```python
from build123d import *

# Parameters (mm, degrees)
SKETCH2_W                  = 20.32
SKETCH2_H                  = 2.41
BOSS_EXTRUDE1_DEPTH        = 8.51
SKETCH5_W                  = 1
SKETCH5_H                  = 1
CUT_EXTRUDE1_DEPTH         = 5
CHAMFER1_SIZE              = 0.5
LPATTERN3_COUNT            = 8
LPATTERN3_PITCH            = 2.54
CHAMFER1_OF_LPATTERN3_SIZE = 0.5
SKETCH11_W                 = 0.64
SKETCH11_H                 = 0.64
BOSS_EXTRUDE2_DEPTH        = 9.92
LPATTERN4_COUNT            = 8
LPATTERN4_PITCH            = 2.54


with BuildPart() as part:
    # Sketch2 → Boss-Extrude1 (new body)
    with BuildSketch(Plane(origin=(0, 0, 0), x_dir=(1, 0, 0), z_dir=(0, 1, 0))):
        with Locations((8.89, 0)):
            Rectangle(SKETCH2_W, SKETCH2_H)
    extrude(amount=BOSS_EXTRUDE1_DEPTH)

    # Sketch5 → Cut-Extrude1 (cut)
    with BuildSketch(Plane(origin=(0, 8.51, 0), x_dir=(1, 0, 0), z_dir=(0, 1, 0))):
        Rectangle(SKETCH5_W, SKETCH5_H)
    cut_extrude1 = extrude(amount=-CUT_EXTRUDE1_DEPTH, mode=Mode.SUBTRACT)

    # Chamfer1
    chamfer1_edges = [part.edges().sort_by_distance(p)[0] for p in [
        (0.5, 8.51, 0),
        (0, 8.51, -0.5),
        (-0.5, 8.51, 0),
        (0, 8.51, 0.5),
    ]]
    chamfer(chamfer1_edges, length=CHAMFER1_SIZE)

    # LPattern3: Cut-Extrude1 ×8
    with Locations(*[(i * LPATTERN3_PITCH, 0, 0) for i in range(1, LPATTERN3_COUNT)]):
        add(cut_extrude1, mode=Mode.SUBTRACT)

    # Chamfer1 of LPattern3
    chamfer1_of_lpattern3_edges = [part.edges().sort_by_distance(p)[0] for p in [
        (3.04, 8.51, 0),
        (2.54, 8.51, -0.5),
        (2.04, 8.51, 0),
        (2.54, 8.51, 0.5),
        (5.58, 8.51, 0),
        (5.08, 8.51, -0.5),
        (4.58, 8.51, 0),
        (5.08, 8.51, 0.5),
        (8.12, 8.51, 0),
        (7.62, 8.51, -0.5),
        (7.12, 8.51, 0),
        (7.62, 8.51, 0.5),
        (10.66, 8.51, 0),
        (10.16, 8.51, -0.5),
        (9.66, 8.51, 0),
        (10.16, 8.51, 0.5),
        (13.2, 8.51, 0),
        (12.7, 8.51, -0.5),
        (12.2, 8.51, 0),
        (12.7, 8.51, 0.5),
        (15.74, 8.51, 0),
        (15.24, 8.51, -0.5),
        (14.74, 8.51, 0),
        (15.24, 8.51, 0.5),
        (18.28, 8.51, 0),
        (17.78, 8.51, -0.5),
        (17.28, 8.51, 0),
        (17.78, 8.51, 0.5),
    ]]
    chamfer(chamfer1_of_lpattern3_edges, length=CHAMFER1_OF_LPATTERN3_SIZE)

    # Sketch11 → Boss-Extrude2 (add)
    with BuildSketch(Plane.XZ):
        Rectangle(SKETCH11_W, SKETCH11_H)
    boss_extrude2 = extrude(amount=BOSS_EXTRUDE2_DEPTH)

    # Sketch13 → Loft1 section 0
    with BuildSketch(Plane.XZ.offset(9.92)):
        with BuildLine():
            Line((0.32, -0.32), (0.32, 0.32))
            Line((0.32, 0.32), (-0.32, 0.32))
            Line((-0.32, 0.32), (-0.32, -0.32))
            Line((-0.32, -0.32), (0.32, -0.32))
        make_face()
    # Sketch14 → Loft1 section 1
    with BuildSketch(Plane(origin=(0, -10.49, 0), x_dir=(-1, 0, 0), z_dir=(0, -1, 0))):
        with BuildLine():
            Line((-0.22, 0.22), (0.22, 0.22))
            Line((0.22, 0.22), (0.22, -0.22))
            Line((0.22, -0.22), (-0.22, -0.22))
            Line((-0.22, -0.22), (-0.22, 0.22))
        make_face()
    loft1 = loft()

    # LPattern4: Boss-Extrude2, Loft1 ×8
    with Locations(*[(i * LPATTERN4_PITCH, 0, 0) for i in range(1, LPATTERN4_COUNT)]):
        add(boss_extrude2)
        add(loft1)


solid = part.part
```
Source: CAD feature listing. Evaluate the final solid. Frame: model axes, mm. A direction names the side the tool comes from. Coordinates: 2 decimals unless noted, no trailing zeros. Loops run counter-clockwise (first coordinate to the right, second up) from the corner with the lowest first, then second, coordinate; pieces in that order, holes last. Notation, with made-up numbers: M 65.5,15 L 100.5,15 A32 cw 100.5,41 Z; hole C 30.5,4 d8. An arc over 180 degrees is marked long. Use a Markdown table: item, result. Add a question column.
Q1. Draft query along Z for faces 1 (the flat face through (19.05, 4, 0)), 2 (the flat face through (10, 3.51, 0)), 3 (the flat face through (12.2, 6, 0)), 4 (the flat face through (9, 4, -1.205)). Return one class per face: pulls with the +Z half, pulls with the -Z half, needs draft (parallel to the pull), parting line crosses it, or undercut.
Q2. Section query C-C, the plane x = 14. Return loops of the section in (y, z) (3 decimals).
Q3. Access query for faces 5 (the flat face through (9, 8.51, 0)), 6 (the flat face through (13, 6, 0.5)). Directions: +Z, -Z, +X, -X, +Y, -Y. A direction counts if a zero-diameter tool reaches every point of the face in a straight line with its end or side. Return the directions, or none.
Q4. Section query A-A, the plane y = -5. State how many separate pieces and enclosed holes the cut face has, and give its area (3 significant figures).
Q5. Material intervals for L1, parallel to Y at x = 10.25, z = -0.15; L2, parallel to Z at x = 0, y = -3; L3, parallel to Y at x = 16.25, z = -0.9, sorted ascending.
Q6. First-contact query: pin 1 (6 mm diameter, centred on x = 7, y = -2, fed in from +Z) (3 decimals); pin 2 (0.7 mm diameter, centred on y = -6, z = 0, fed in from -X); pin 3 (1.2 mm diameter, centred on x = 9, z = 0, fed in from -Y); pin 4 (3 mm diameter, centred on x = 1.5, y = -7, fed in from +Z). Flat tips, straight axial feed; report the tip coordinate or a pass-through.
Result:
| question | item | result |
|---|---|---|
| 1 | face 1 | needs draft |
| 1 | face 2 | undercut |
| 1 | face 3 | undercut |
| 1 | face 4 | pulls with the -Z half |
| 2 | outline | M 0,-1.205 L 8.51,-1.205 L 8.51,1.205 L 0,1.205 Z |
| 3 | face 5 | +Z, -Z, +X, -X, +Y |
| 3 | face 6 | +Y |
| 4 | separate pieces | 8 |
| 4 | enclosed holes | 0 |
| 4 | area | 3.28 mm2 |
| 5 | L1 | y = -10.49 to 3.51 |
| 5 | L2 | z = -0.32 to 0.32 |
| 5 | L3 | y = 0 to 8.51 |
| 6 | pin 1 | stops at z = 1.205 |
| 6 | pin 2 | stops at x = -0.32 |
| 6 | pin 3 | stops at y = 0 |
| 6 | pin 4 | stops at z = 0.32 |
